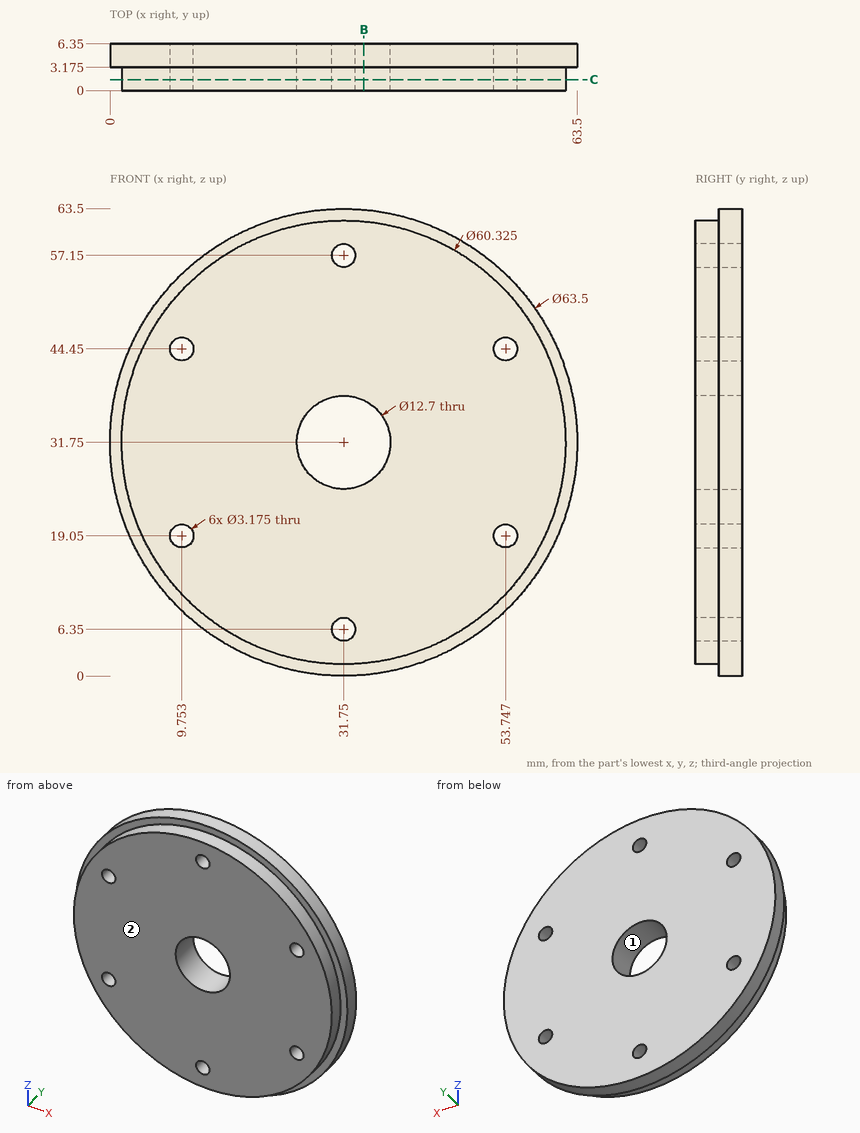
Input: dimensioned drawing with shaded views. Units: mm. Origin: part minimum x, y, z. Round coordinates to 2 decimals unless told otherwise and drop trailing zeros. Loops run counter-clockwise (first coordinate to the right, second up) from the corner with the lowest first, then second, coordinate; pieces in that order, holes last. Notation, with made-up numbers: (49, 7.5) -> (94, 7.5) arc R28 cw to (94, 45.5) -> close; hole circle Ø6 at (84, -16). An arc over 180 degrees is marked (long way). One line per item, written item: value.
(1) Pin query (flat end, axial travel): pin 1 (1.5 mm diameter, centred on x = 20.5, y = 3.5, fed in from -Z); pin 2 (1 mm diameter, centred on y = 1.5, z = 37, fed in from -X); pin 3 (2 mm diameter, centred on x = 8, y = 4.5, fed in from -Z). Return the tip coordinate at first contact, or that it passes through.
Geometry check:
pin 1: z = 1.79
pin 2: x = 1.96
pin 3: z = 9.6
(2) Mould query, pull axis Z, two halves, no side actions, for the marked faces 1 and 2. Classes: pulls with the +Z half, pulls with the -Z half, needs draft (parallel to the pull), parting line crosses it, or undercut.
Geometry check:
face 1: undercut
face 2: needs draft
(3) Section C-C (y = 1.5). Give the number of separate pieces and of enclosed holes in the cut face, plus the area to 3 significant figures.
Geometry check:
separate pieces: 1
enclosed holes: 7
area: 2,680 mm2
(4) Section B-B (x = 34.5). Return the cut outline in (y, z) (3 decimals).
Geometry check:
outline: (0, 1.713) -> (3.175, 1.713) -> (3.175, 0.119) -> (6.35, 0.119) -> (6.35, 26.026) -> (0, 26.026) -> close; (0, 37.474) -> (6.35, 37.474) -> (6.35, 63.381) -> (3.175, 63.381) -> (3.175, 61.787) -> (0, 61.787) -> close
(5) Material intervals for line 1 (X direction, y = 3.25, z = 31.75); line 2 (X direction, y = 2.75, z = 44.45); line 3 (Z direction, x = 54, y = 2.5), sorted ascending. Write a range as [from, to].
Geometry check:
line 1: [0, 25.4], [38.1, 63.5]
line 2: [4.39, 8.17], [11.34, 52.16], [55.33, 59.11]
line 3: [11.39, 17.48], [20.62, 42.88], [46.02, 52.11]
